The drawing under review shows one solid part. Ordinate dimensions are in mm from its lowest x, y, z. A direction names the side the tool comes from. Coordinates: 2 decimals unless noted, no trailing zeros. Loops run counter-clockwise (first coordinate to the right, second up) from the corner with the lowest first, then second, coordinate; pieces in that order, holes last. Notation, with made-up numbers: M 3.5,46 L 17.5,46 A20 cw 17.5,79 Z; hole C 64,21.25 d6. An arc over 180 degrees is marked long. Return JSON: item names as keys, results as strings.
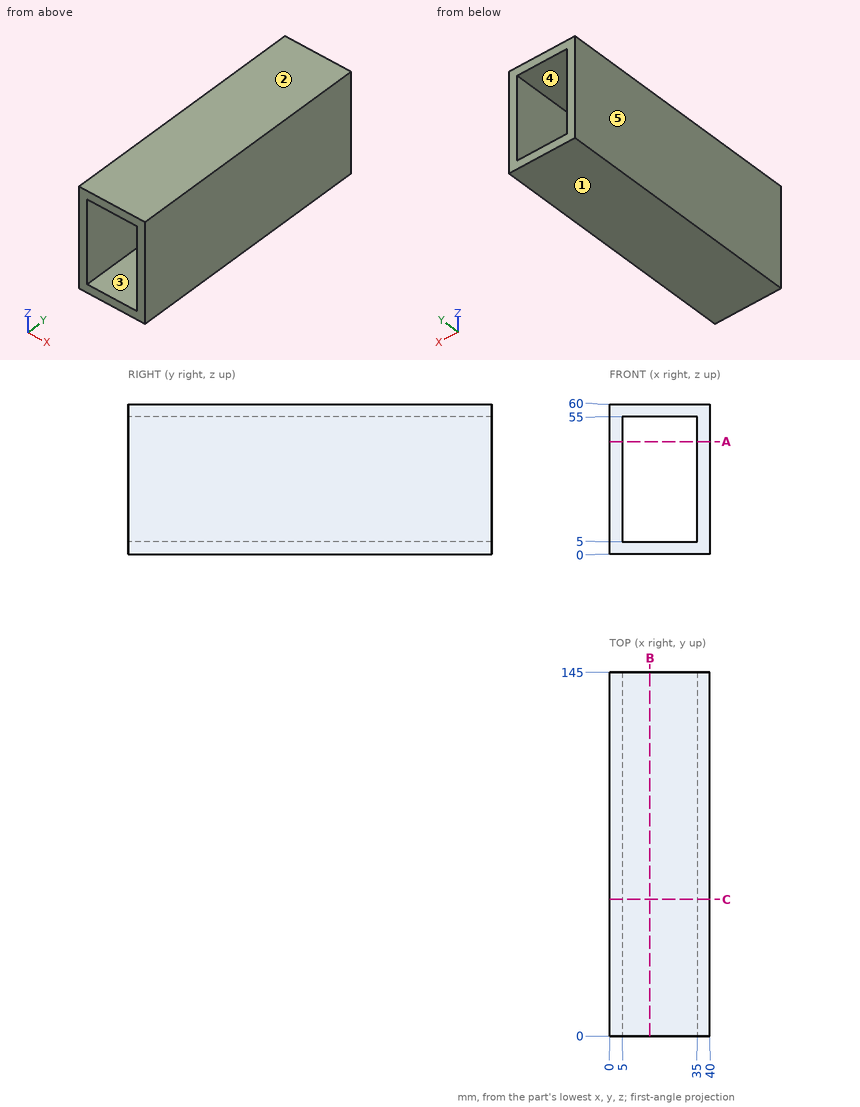
1. The part is to be moulded in two halves that separate along Z. For the marked faces 1, 2 and 3, say which applies: released by +Z, released by -Z, zero draft, split by the parting line, or undercut.
Check values:
{"face 1": "released by -Z", "face 2": "released by +Z", "face 3": "undercut"}
2. Machinability: for the marked faces 4 and 5, which of the approach directions +Z, -Z, +X, -X, +Y, -Y give a long, thin tool a straight path to every point of the face, cutting with its end or side? Answer none if there is none.
Check values:
{"face 4": "+Y, -Y", "face 5": "+Z, -Z, -X, +Y, -Y"}
3. Add section B-B on x = 16. Give the boundary of the cut face in (y, z).
Check values:
{"outline": "M 0,0 L 145,0 L 145,5 L 0,5 Z; M 0,55 L 145,55 L 145,60 L 0,60 Z"}
4. Add section A-A on z = 45. Give the boundary of the cut face in (x, y), plus the area to 3 significant figures.
Check values:
{"outline": "M 0,0 L 5,0 L 5,145 L 0,145 Z; M 35,0 L 40,0 L 40,145 L 35,145 Z", "area": "1,450 mm²"}
5. Add section C-C on y = 54.5. Give the boundary of the cut face in (x, z).
Check values:
{"outline": "M 0,0 L 40,0 L 40,60 L 0,60 Z; hole M 5,5 L 35,5 L 35,55 L 5,55 Z"}
6. To check wall thickness, follow line 1 (Z direction, x = 22, y = 114); line 2 (X direction, y = 35, z = 46). State the ranges of each line that lie inside material, in increasing order.
Check values:
{"line 1": "0 to 5, 55 to 60", "line 2": "0 to 5, 35 to 40"}
